```python
from build123d import *

# Parameters (mm, degrees)
F1_DEPTH = 58.166
F2_R     = 17.879779
F3_DEPTH = 52.592631
F5_DEPTH = 27.403686


with BuildPart() as f1:
    # F0 (on Front) → F1 (new body)
    with BuildSketch(Plane.XZ):
        Polygon((0, -40.496975), (0, 0), (25.188945, 0), (25.188945, 75.828001), (-27.402686, 75.828001), (-27.402686, -40.496975), align=None)
    extrude(amount=F1_DEPTH)

    # F2 (on face) → F3 (cut, through all)
    with BuildSketch(Plane.YZ.offset(25.188945)):
        with Locations((-29.593647, 39.162569)):
            Circle(F2_R)
    extrude(amount=-F3_DEPTH, mode=Mode.SUBTRACT)

    # F4 (on face) → F5 (cut, through all)
    with BuildSketch(Plane.YZ):
        with BuildLine():
            Line((-54.177677, -40.496975), (-3.988323, -40.496975))
            ThreePointArc((-3.988323, -40.496975), (-29.083, -15.402298), (-54.177677, -40.496975))
        make_face()
    extrude(amount=-F5_DEPTH, mode=Mode.SUBTRACT)


solid = f1.part
```
Model file for the job. Use its own axes, mm. A direction names the side the tool comes from. Give positions to 0.01 mm unless a question says otherwise; leave off trailing zeros. Loops run counter-clockwise (first coordinate to the right, second up) from the corner with the lowest first, then second, coordinate; pieces in that order, holes last. Notation, with made-up numbers: (84.25, 46.25) - (93.25, 46.25) arc R13 ccw to (93.25, 55.25) - close; hole circle Ø4 at (22, 6). An arc over 180 degrees is marked (long way). One line per item, written item: value. Start each with the question number.
1. Slice it at C-C (x = -12). List the corners of the cut face in (y, z), plus the area to 3 significant figures.
2. Pin check, flat tip, straight feed: pin 1 (20 mm diameter, centred on x = 17.5, y = -24.5, fed in from -Z). Stop position of the tip, or through.
3. Pull direction Y, two halves, no side cores. Call faces 3 (the cylindrical face through (-13.51, -28.53, -15.41)), 4 (the flat face through (-1, -58.166, 31)), 5 (the flat face through (12, -29, 0)): pulls with the +Y half, pulls with the -Y half, needs draft (parallel to the pull), parting line crosses it, or undercut.
4. Slice it at D-D (z = -12). List the corners of the cut face in (x, y).
5. Which spindle directions (+Z, -Z, +X, -X, +Y, -Y) get a long thin tool onto all of the face, cutting with end or side? Do faces 1 (the flat face through (0, -29, -12)), 2 (the flat face through (-14, -56, -40.497)). Say none if no direction does.
6. Probe L1, parallel to Z at x = -6.5, y = -22; L2, parallel to Z at x = 15, y = -48; L3, parallel to Z at x = -22, y = -17.5. List the from-to ranges inside material, lowest first. Write a range as from..to.
7. Slice it at B-B (z = 38). List the corners of the cut face in (x, y), plus the area to 3 significant figures.
8. Slice it at A-A (y = -29.5). List the corners of the cut face in (x, z).
Solution:
1. outline: (-58.17, -40.5) - (-54.18, -40.5) arc R25.09 cw to (-3.99, -40.5) - (0, -40.5) - (0, 75.83) - (-58.17, 75.83) - close; hole circle Ø35.76 at (-29.59, 39.16)
1. area: 4,770 mm^2
2. pin 1: stops at z = 0
3. face 3: undercut
3. face 4: pulls with the -Y half
3. face 5: needs draft
4. outline: (-27.4, -58.17) - (0, -58.17) - (0, 0) - (-27.4, 0) - close
5. face 1: -Z, +X, +Y, -Y
5. face 2: -Z, +X, -X, +Y, -Y
6. L1: z = -16.42..22.98, 55.35..75.83
6. L2: z = 0..75.83
6. L3: z = -18.24..25.99, 52.33..75.83
7. outline: (-27.4, -58.17) - (25.19, -58.17) - (25.19, -47.44) - (-27.4, -47.44) - close; (-27.4, -11.75) - (25.19, -11.75) - (25.19, 0) - (-27.4, 0) - close
7. area: 1,180 mm^2
8. outline: (-27.4, -15.41) - (0, -15.41) - (0, 0) - (25.19, 0) - (25.19, 21.28) - (-27.4, 21.28) - close; (-27.4, 57.04) - (25.19, 57.04) - (25.19, 75.83) - (-27.4, 75.83) - close
